from build123d import *

# Parameters (mm, degrees)
SKETCH_1_R      = 1
EXTRUDE_1_DEPTH = 0.5
FILLET_1_R      = 1


with BuildPart() as part:
    # 草图1 → 凸台-拉伸1 (new, symmetric)
    with BuildSketch(Plane(origin=(0, 0, 0), x_dir=(1, 0, 0), z_dir=(0, 1, 0))):
        with BuildLine():
            Line((-1.25, -13.341570372), (-1.25, -9.16515139))
            ThreePointArc((-1.25, -9.16515139), (0, 9.25), (1.25, -9.16515139))
            Line((1.25, -9.16515139), (1.25, -13.341570372))
            ThreePointArc((1.25, -13.341570372), (4.374478114, -12.665857303), (7.25, -11.269316749))
            Line((7.25, -11.269316749), (7.25, -7.932325267))
            ThreePointArc((7.25, -7.932325267), (0, 11.92), (-7.25, -7.932325267))
            Line((-7.25, -7.932325267), (-7.25, -11.269316749))
            ThreePointArc((-7.25, -11.269316749), (-4.374478114, -12.665857303), (-1.25, -13.341570372))
        make_face()
        with Locations(Location((-4.25, -10.362311518, 0), (0, 0, 270))):
            Circle(SKETCH_1_R, mode=Mode.SUBTRACT)
        with Locations(Location((4.25, -10.362311518, 0), (0, 0, 90))):
            Circle(SKETCH_1_R, mode=Mode.SUBTRACT)
    extrude(amount=EXTRUDE_1_DEPTH, both=True)

    # 圆角1
    fillet_1_edges = [part.edges().sort_by_distance(p)[0] for p in [
        (7.25, 0, 7.932325267),
        (7.25, 0, 11.269316749),
        (1.25, 0, 13.341570372),
        (1.25, 0, 9.16515139),
        (-1.25, 0, 9.16515139),
        (-1.25, 0, 13.341570372),
        (-7.25, 0, 11.269316749),
        (-7.25, 0, 7.932325267),
    ]]
    fillet(fillet_1_edges, radius=FILLET_1_R)


solid = part.part
CAD build for the part. Positions are in the model's coordinates, mm. A direction names the side the tool comes from. Round coordinates to 2 decimals unless told otherwise and drop trailing zeros. Write each loop counter-clockwise with the first axis right and the second up, starting at its lowest first coordinate (ties: lowest second). Pieces come first, ordered by that corner, then holes.
(1) Mould opens along Z. For faces 1 (the face through (-3.9, 0, 11.3)), 2 (the face through (1.62, 0.01, 12.97)), 3 (the face through (-5, -0.5, -8)) say: pulls with the +Z half, pulls with the -Z half, needs draft (parallel to the pull), parting line crosses it, or undercut.
(2) Slice it at B-B, the plane y = 0.15. Write the cut outline in (x, z), and give its area (3 significant figures).
(3) Drop flat-ended pins along their axis: P1, Ø12, axis at x = 0, z = -3, coming from the -Y side; P2, Ø0.5, axis at y = 0, z = 9.5, coming from the +X side. Give the stop position or say it passes through.
(4) Slice it at C-C, the plane x = 4.25. Write the cut outline in (y, z), and give its area (3 significant figures).
(5) Probe line 1 along Z through (x, y) = (4.25, -0.2); line 2 along X through (y, z) = (0.4, 9.75); line 3 along X through (y, z) = (0.3, -5.5). List the from-to ranges inside material, lowest first.
(6) Slice it at D-D, the plane z = -6.5. Write the cut outline in (x, y).
(7) 3-axis set-ups, long thin cutter, end or side, ignore diameter. For faces 4 (the face through (-7.25, 0, 10)), 5 (the face through (1.25, 0, 11)), 6 (the face through (7.25, 0, 10)): which of +Z, -Z, +X, -X, +Y, -Y reach the whole face in a straight line?
(8) Slice it at A-A, the plane z = 8.75. Write the cut outline in (x, y), and give its area (3 significant figures).
From the geometry:
1. face 1: undercut
1. face 2: pulls with the +Z half
1. face 3: needs draft
2. outline: (-7.58, 7.65) arc R11.25 ccw (long way) to (7.58, 7.65) arc R1 cw to (7.25, 8.39) - (7.25, 10.71) arc R1 ccw to (6.75, 11.57) arc R13.4 ccw to (2.43, 13.18) arc R1 ccw to (1.25, 12.19) - (1.25, 10) arc R1 ccw to (2.03, 9.02) arc R9.25 cw (long way) to (-2.03, 9.02) arc R1 ccw to (-1.25, 10) - (-1.25, 12.19) arc R1 ccw to (-2.43, 13.18) arc R13.4 ccw to (-6.75, 11.57) arc R1 ccw to (-7.25, 10.71) - (-7.25, 8.39) arc R1 cw to start; hole circle Ø2 at (-4.25, 10.36); hole circle Ø2 at (4.25, 10.36)
2. area: 154 mm2
3. P1: passes through
3. P2: stops at x = 7.25
4. outline: (-0.5, -11.09) - (0.5, -11.09) - (0.5, -8.22) - (-0.5, -8.22) - close; (-0.5, 8.22) - (0.5, 8.22) - (0.5, 9.36) - (-0.5, 9.36) - close; (-0.5, 11.36) - (0.5, 11.36) - (0.5, 12.71) - (-0.5, 12.71) - close
4. area: 5.36 mm2
5. line 1: z = -11.09 to -8.22, 8.22 to 9.36, 11.36 to 12.71
5. line 2: x = -7.25 to -5.04, -3.46 to -1.28, 1.28 to 3.46, 5.04 to 7.25
5. line 3: x = -10.16 to -7.44, 7.44 to 10.16
6. outline: (-9.62, -0.5) - (-6.58, -0.5) - (-6.58, 0.5) - (-9.62, 0.5) - close; (6.58, -0.5) - (9.62, -0.5) - (9.62, 0.5) - (6.58, 0.5) - close
7. face 4: +Z, -X, +Y, -Y
7. face 5: +Z, +Y, -Y
7. face 6: +Z, +X, +Y, -Y
8. outline: (-7.25, -0.5) - (-3, -0.5) - (-3, 0.5) - (-7.25, 0.5) - close; (3, -0.5) - (7.25, -0.5) - (7.25, 0.5) - (3, 0.5) - close
8. area: 8.50 mm2
